Verification items for the finished model (mm, model axes). Face numbers are marked on the shaded views. A direction names the side the tool comes from. Round coordinates to 2 decimals unless told otherwise and drop trailing zeros. Write each loop counter-clockwise with the first axis right and the second up, starting at its lowest first coordinate (ties: lowest second). Pieces come first, ordered by that corner, then holes. Notation, with made-up numbers: M -22.75,-8.5 L 26.25,-8.5 A25 ccw 26.25,23.5 Z; hole C 3.5,-8.75 d5. An arc over 180 degrees is marked long. Answer in a Markdown table with one row per item. Add a question column.
1. Sectioned sample at A-A on x = 5. Record the cut outline in (y, z), plus the area to 3 significant figures.
2. Go/stop test with flat-tipped pins: pin 1 Ø2 at (x, z) = (6, 7.5) entering from +Y; pin 2 Ø6 at (x, y) = (3.5, 5.5) entering from -Z; pin 3 Ø4 at (x, z) = (7.5, 4.5) entering from +Y; pin 4 Ø4 at (y, z) = (0, 6) entering from -X. Record where each tip stops, or that it passes through.
3. Sectioned sample at B-B on x = 10.5. Record the cut outline in (y, z), plus the area to 3 significant figures.
4. Sectioned sample at C-C on x = 2. Record the cut outline in (y, z).
5. Material ranges on probe 1 along Y at (x, z) = (10.25, 0); probe 2 along Z at (x, y) = (3.25, 0), recorded low to high.
6. Draft check along Z on the marked faces 1, 2, 3 and 4. Enter one of: pulls with the +Z half, pulls with the -Z half, needs draft (parallel to the pull), parting line crosses it, or undercut.
7. Set-up check for the marked faces 5, 6 and 7: record each of +Z, -Z, +X, -X, +Y, -Y from which the full face is reachable in a straight line by a thin tool's end or side.
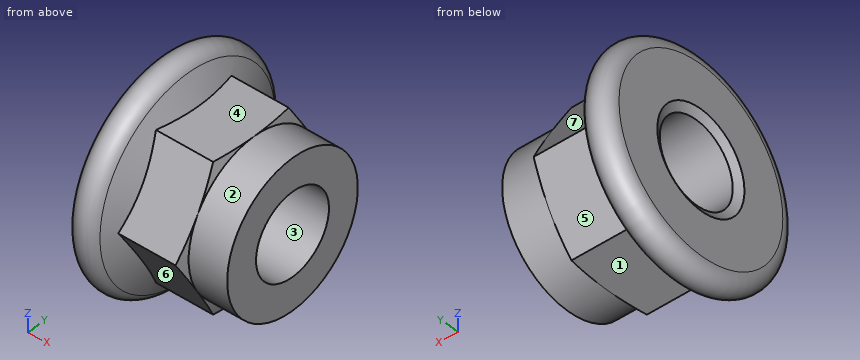
Autodesk Inventor part; units mm, degrees
ref_plane "Work Plane1" through (33.6561, 0, 0) normal (0, 0, -1) x (-1, 0, 0)
ref_plane "YZ Plane" through (0, 0, 0) normal (1, 0, 0) x (0, 1, 0)
ref_plane "XZ Plane" through (0, 0, 0) normal (0, 1, 0) x (-1, 0, 0)
sketch "Szkic1" plane through (0, 0, 0) normal (0, 0, 1) x (1, 0, 0)
  line L0 (-3.0053, 0) -> (16.2509, 0)
  line L1 (4.0411, 7.5) -> (2.8595, 10.0339)
  line L2 (4.0411, 7.5) -> (13.5, 7.5) construction
  line L3 (13.5, 7.5) -> (13.5, 0) construction
  arc A0 (2.8595, 10.0339) -> (0, 9.4) centre (1.5, 9.4) ccw
  line L4 (4.0411, 7.5) -> (4.0411, 0)
  line L5 (0, -2.2363) -> (0, 13.4177)
  point P0 (0, 0)
  dimension "d1" = 15
  dimension "d3" = 21.8
  dimension "d4" = 1.5
  dimension "d16" = 13.5
  dimension "d17" = 25
revolve "Pierścień" add sketch "Szkic1" angle 360 about axis through (-10, 0, 0) along (1, 0, 0)
sketch "Szkic2" plane through (0, 0, 0) normal (-1, 0, 0) x (0, 0, 1)
  circle A0 centre (0, 0) radius 4.9
  line L0 (-7.5, -4.3301) -> (-7.5, 4.3301)
  line L1 (-7.5, 4.3301) -> (0, 8.6603)
  line L2 (0, 8.6603) -> (7.5, 4.3301)
  line L3 (7.5, 4.3301) -> (7.5, -4.3301)
  line L4 (7.5, -4.3301) -> (0, -8.6603)
  line L5 (0, -8.6603) -> (-7.5, -4.3301)
  circle A1 centre (0, 0) radius 9.4
  dimension "d5" = 17.3205
extrude "Bryła" add sketch "Szkic2" against normal blind 9.6 contours A0 | L0 L1 L2 L3 L4 L5
sketch "Szkic3" plane through (9.6, 0, 0) normal (1, 0, 0) x (0, 0, -1)
  circle A0 centre (0, 0) radius 7.5
  dimension "d19" = 15
extrude "Zamek" add sketch "Szkic3" along normal blind 3.9
sketch "Szkic4" plane through (0, 0, 0) normal (-1, 0, 0) x (0, 0, 1)
  circle A0 centre (0, 0) radius 4.9
  circle A1 centre (0, 0) radius 9.4
hole "Gwint" at (0, 0, 0) direction (1, 0, 0) diameter 8.376 end through all
sketch "Szkic5" plane through (0, 0, 0) normal (0, 0, 1) x (1, 0, 0)
  line L0 (3.5, 8.6603) -> (9.6, 8.6603)
  line L1 (9.6, 4.3301) -> (9.6, 8.6603)
  line L2 (0, -9.4) -> (0, 9.4)
  line L3 (-1.92, 0) -> (11.52, 0)
  line L4 (9.2891, 8.6603) -> (9.6, 7.5)
  dimension "d9" = 15
  dimension "d10" = 15
revolve "Faza1" cut sketch "Szkic5" angle 360 about axis through (-10, 0, 0) along (1, 0, 0)
chamfer "Faza2" distance 0.8119 angle 30 1 edges at (0, 0, -4.188) measured on face at (0, 7.5614, -0.9181)
ref_plane "Work Plane1" through (33.6561, 0, 0) normal (0, 0, -1) x (-1, 0, 0)
equation "\"d1\" = SW"
equation "\"d3\" = LADI"
equation "\"d4\" = PHH"
equation "\"d16\" = KOH"
equation "\"d17\" = KEWI"
equation "\"d5\" = 1.1547 * SW"
equation "\"d6\" = KOH1"
equation "\"d19\" = SD2"
equation "\"d11\" = KOH - KOH1"
equation "\"d9\" = ANG1"
equation "\"d10\" = SW0"
equation "\"d13\" = -0.5 * GD1 + 0.5 * NND"
equation "\"d57\" = -0.5 * GD1 + 0.5 * NND"
equation "\"ANG1\" = 15deg"
equation "\"KEWI\" = 25deg"
equation "\"LADI\" = 21.8"
equation "\"SW\" = 15"
equation "\"PHH\" = RR"
equation "\"KOH\" = 13.5"
equation "\"SW0\" = SW"
equation "\"d0\" = LADI"
equation "\"d2\" = PHH"
equation "\"KOH1\" = 9.6"
equation "\"SD2\" = SW"
equation "\"GUL\" = 0.541266 * PTC"
equation "\"RR\" = 1.5"
equation "\"TOA\" = 30deg"
equation "\"PTC\" = 1.5"
equation "\"GAL\" = 0.541266 * PTC"
equation "\"E0\" = 1.155 * SW"
properties part number "DIN 6926 - M10" material "Stal, miękka"
Geometry check:
| question | item | result |
|---|---|---|
| 1 | outline | M -8.66,0 L -4.33,-7.5 L 4.33,-7.5 L 8.66,0 L 4.33,7.5 L -4.33,7.5 Z; hole C 0,0 d8.38 |
| 1 | area | 140 mm2 |
| 2 | pin 1 | stops at y = 4.91 |
| 2 | pin 2 | stops at z = -10.44 |
| 2 | pin 3 | stops at y = 7.22 |
| 2 | pin 4 | stops at x = 0 |
| 3 | outline | C 0,0 d15; hole C 0,0 d8.38 |
| 3 | area | 122 mm2 |
| 4 | outline | C 0,0 d21.63; hole C 0,0 d8.38 |
| 5 | probe 1 | y = -7.5 to -4.19, 4.19 to 7.5 |
| 5 | probe 2 | z = -9.2 to -4.19, 4.19 to 9.2 |
| 6 | face 1 | pulls with the -Z half |
| 6 | face 2 | parting line crosses it |
| 6 | face 3 | undercut |
| 6 | face 4 | pulls with the +Z half |
| 7 | face 5 | -Z, +X, +Y |
| 7 | face 6 | -Z, +X, -Y |
| 7 | face 7 | +Z, +X, +Y |
